Drawing for the job (mm, zero at the part's lowest x, y, z). A direction names the side the tool comes from. Give positions to 0.01 mm unless a question says otherwise; leave off trailing zeros. Order: outer loops, then holes, each group sorted by start corner. A loop starts at its lowest first (then second) coordinate and runs counter-clockwise, first axis right, second up. Notation, with made-up numbers: (-4.5, 65.25) - (51.5, 65.25) arc R30 cw to (51.5, 91.25) - close; hole circle Ø7 at (-34, 61.5). An arc over 180 degrees is marked (long way). One line per item, written item: value.
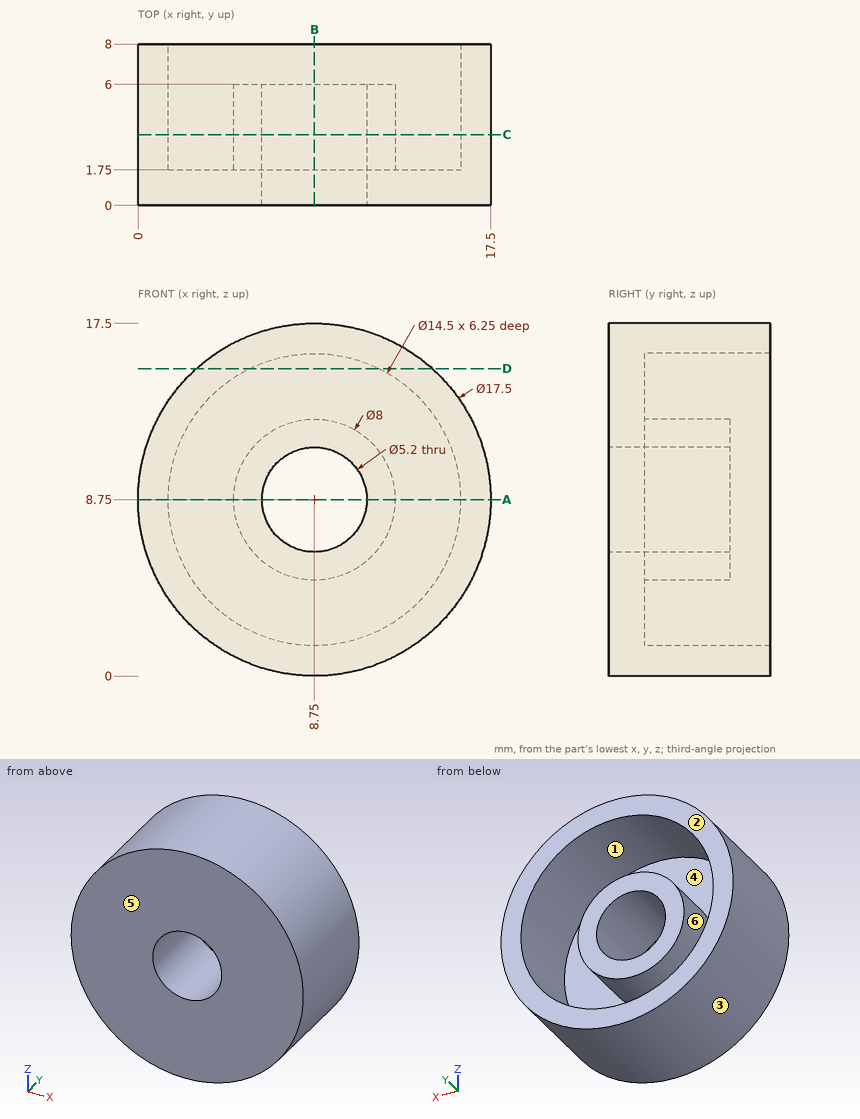
(1) Pin check, flat tips, straight feed: P1, Ø7, axis at x = 6, z = 7, coming from the +Y side; P2, Ø1.5, axis at x = 15, y = 3, coming from the -Z side; P3, Ø1, axis at y = 1.5, z = 5, coming from the +X side. Stop position of each tip, or through.
Completed:
P1: y = 6
P2: z = 1.94
P3: x = 16.87
(2) Slice it at D-D, the plane z = 15.25. Give the cut face in (x, y).
Completed:
outline: (2.89, 0) - (14.61, 0) - (14.61, 8) - (11.96, 8) - (11.96, 1.75) - (5.54, 1.75) - (5.54, 8) - (2.89, 8) - close
(3) Slice it at B-B, the plane x = 8.75. Give the cut face in (y, z), and give its area (3 significant figures).
Completed:
outline: (0, 0) - (8, 0) - (8, 1.5) - (1.75, 1.5) - (1.75, 4.75) - (6, 4.75) - (6, 6.15) - (0, 6.15) - close; (0, 11.35) - (6, 11.35) - (6, 12.75) - (1.75, 12.75) - (1.75, 16) - (8, 16) - (8, 17.5) - (0, 17.5) - close
area: 52.2 mm²
(4) Pull direction X, two halves, no side cores. Call the marked faces 1, 2, 3 and 4: +X half, -X half, draft (parallel to the pull), parting line (faces both ways), or undercut.
Completed:
face 1: undercut
face 2: draft
face 3: parting line
face 4: undercut
(5) Drill centre lines: line 1 (Z direction, x = 8.75, y = 5.5); line 2 (X direction, y = 2.25, z = 9); line 3 (Z direction, x = 12.25, y = 5). Where is each one in solid material? Low to high.
Completed:
line 1: 0 to 1.5, 4.75 to 6.15, 11.35 to 12.75, 16 to 17.5
line 2: 0 to 1.5, 4.76 to 6.16, 11.34 to 12.74, 16 to 17.5
line 3: 0.73 to 2.4, 6.81 to 10.69, 15.1 to 16.77
(6) 3-axis set-ups, long thin cutter, end or side, ignore diameter. For the marked faces 5 and 6: which of +Z, -Z, +X, -X, +Y, -Y reach the whole face in a straight line?
Completed:
face 5: +Z, -Z, +X, -X, -Y
face 6: +Y
(7) Slice it at C-C, the plane y = 3.5. Give the cut face in (x, z), and give its area (3 significant figures).
Completed:
outline: circle Ø17.5 at (8.75, 8.75); circle Ø8 at (8.75, 8.75); hole circle Ø14.5 at (8.75, 8.75); hole circle Ø5.2 at (8.75, 8.75)
area: 104 mm²
(8) Slice it at A-A, the plane z = 8.75. Give the cut face in (x, y), and give its area (3 significant figures).
Completed:
outline: (0, 0) - (6.15, 0) - (6.15, 6) - (4.75, 6) - (4.75, 1.75) - (1.5, 1.75) - (1.5, 8) - (0, 8) - close; (11.35, 0) - (17.5, 0) - (17.5, 8) - (16, 8) - (16, 1.75) - (12.75, 1.75) - (12.75, 6) - (11.35, 6) - close
area: 52.2 mm²
